Can you work these out from the drawing? Everything is in mm from the part's minimum corner. Round coordinates to 2 decimals unless told otherwise and drop trailing zeros. Write each loop counter-clockwise with the first axis right and the second up, starting at its lowest first coordinate (ties: lowest second). Pieces come first, ordered by that corner, then holes. Notation, with made-up numbers: (67, 42) -> (123, 42) arc R23 cw to (123, 61) -> close; hole circle Ø6 at (71, -14.5). An arc over 180 degrees is marked (long way). Write item = value, one per line. Start each with the question number.
1) Imagine slicing it at B-B, the plane z = 23. Please give me the cut outline in (x, y).
2) Imagine slicing it at C-C, the plane y = 2.4. Please give me the cut outline in (x, z).
3) Thinking about a two-plate mould opening in Z: for the marked faces 1, 2 and 3, which applies, +Z half, -Z half, draft (parallel to the pull), parting line (faces both ways), or undercut?
4) If I drill on line 1 (X direction, y = 2.75, z = 7), over which ranges is the centre line in solid material (lowest first)?
5) Imagine slicing it at A-A, the plane x = 22.5. Please give me the cut outline in (y, z).
6) Imagine slicing it at D-D, the plane x = 16. Please give me the cut outline in (y, z).
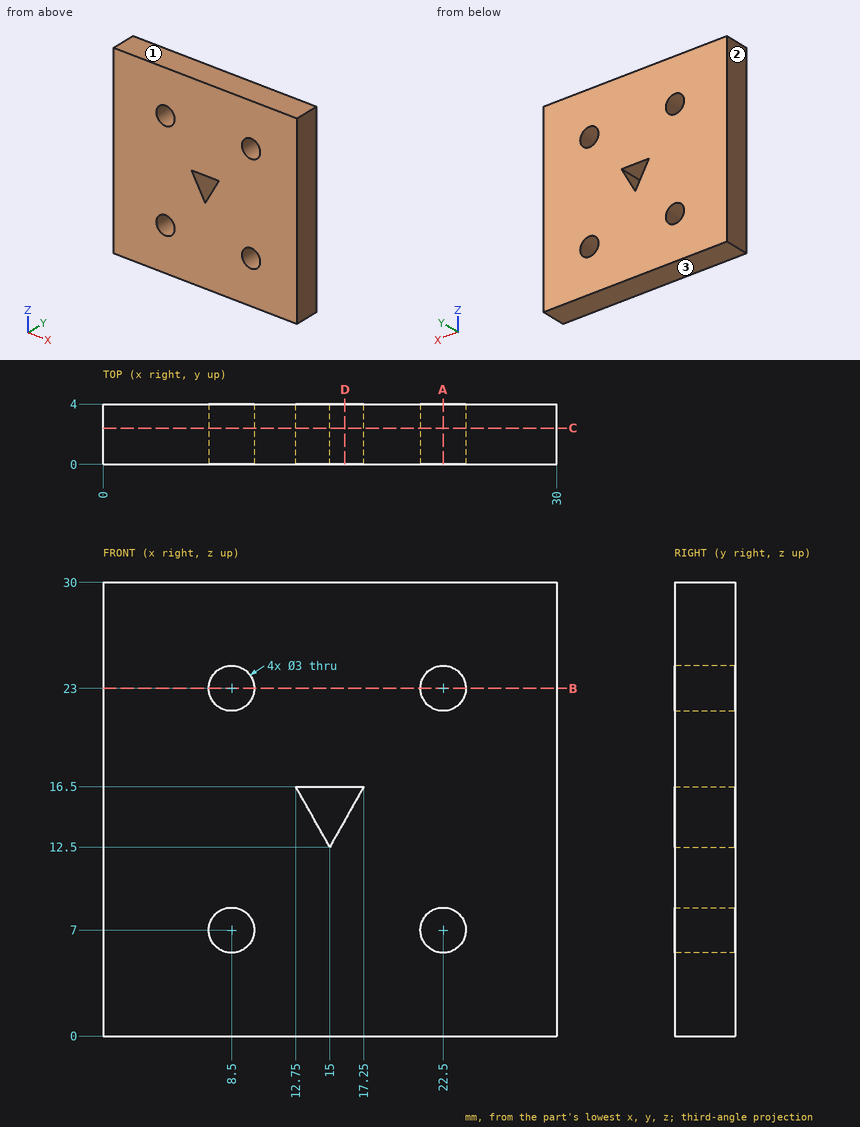
Reported:
q1.outline = (0, 0) -> (7, 0) -> (7, 4) -> (0, 4) -> close; (10, 0) -> (21, 0) -> (21, 4) -> (10, 4) -> close; (24, 0) -> (30, 0) -> (30, 4) -> (24, 4) -> close
q2.outline = (0, 0) -> (30, 0) -> (30, 30) -> (0, 30) -> close; hole circle Ø3 at (8.5, 7); hole circle Ø3 at (8.5, 23); hole (12.75, 16.5) -> (15, 12.5) -> (17.25, 16.5) -> close; hole circle Ø3 at (22.5, 7); hole circle Ø3 at (22.5, 23)
q3.face_1 = +Z half
q3.face_2 = draft
q3.face_3 = -Z half
q4.line_1 = 0 to 7, 10 to 21, 24 to 30
q5.outline = (0, 0) -> (4, 0) -> (4, 5.5) -> (0, 5.5) -> close; (0, 8.5) -> (4, 8.5) -> (4, 21.5) -> (0, 21.5) -> close; (0, 24.5) -> (4, 24.5) -> (4, 30) -> (0, 30) -> close
q6.outline = (0, 0) -> (4, 0) -> (4, 14.28) -> (0, 14.28) -> close; (0, 16.5) -> (4, 16.5) -> (4, 30) -> (0, 30) -> close
